Can you work these out from the drawing? Everything is in mm from the part's minimum corner. A direction names the side the tool comes from. Coordinates: 2 decimals unless noted, no trailing zeros. Loops run counter-clockwise (first coordinate to the right, second up) from the corner with the lowest first, then second, coordinate; pieces in that order, holes last.
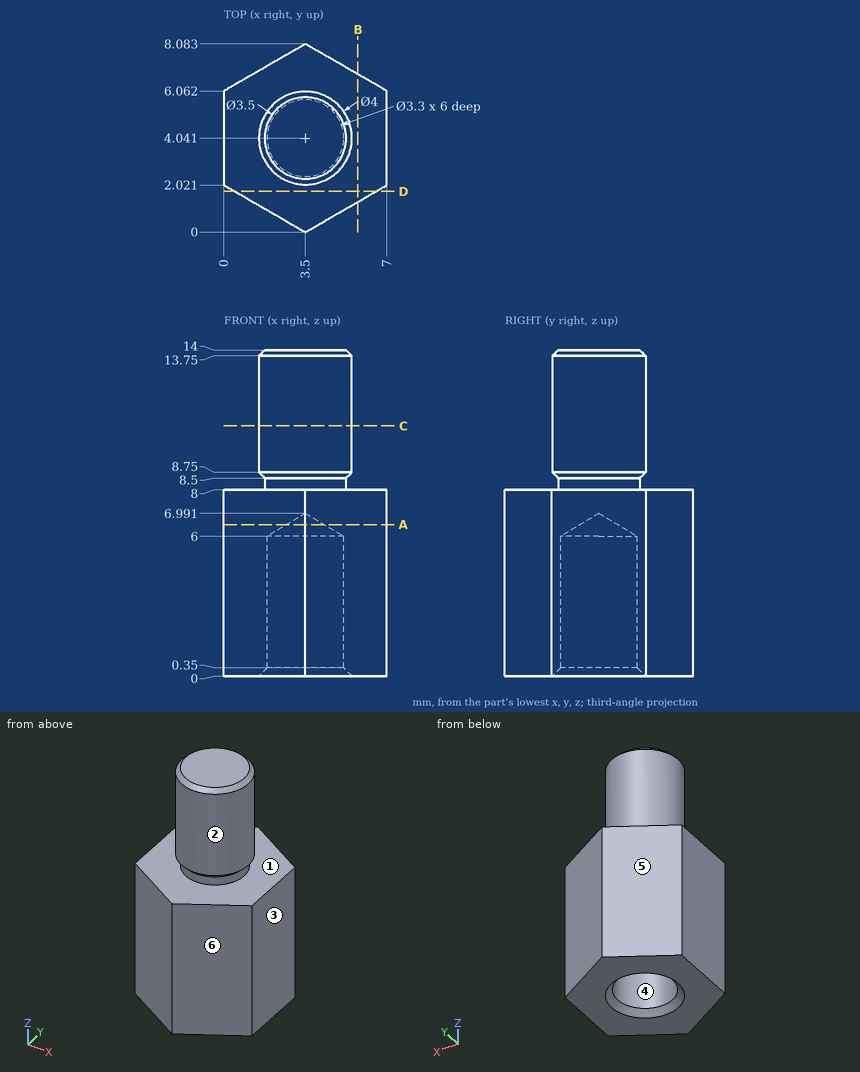
1) Imagine slicing it at C-C on z = 10.75. List the corners of the cut face in (x, y) for me, plus the area to 3 significant figures.
2) Imagine slicing it at A-A on z = 6.5. List the corners of the cut face in (x, y) for me (1 decimal).
3) Imagine slicing it at B-B on x = 5.75. List the corners of the cut face in (y, z) for me.
4) Imagine slicing it at D-D on y = 1.75. List the corners of the cut face in (x, z) for me.
5) For the marked faces 1, 2 and 3, which set-ups out of +Z, -Z, +X, -X, +Y, -Y let a thin tool reach every point of the face, with its end or its side?
6) If I drill on L1, parallel to Z at x = 6.5, y = 4.25; L2, parallel to Y at x = 3, z = 4.5 (1 decimal); L3, parallel to X at y = 4, z = 6.5 (1 decimal), over which ranges is the centre line in solid material (lowest first)?
7) We'd pull the mould along Y, two halves only. Please class the marked faces 4, 5 and 6: released by +Y, released by -Y, zero draft, split by the parting line, or undercut.
8) Will these pins go through, and if not, where does the flat tip stop? pin 1 (3 mm diameter, centred on y = 1, z = 12.5, fed in from +X) (1 decimal); pin 2 (1.1 mm diameter, centred on x = 3, y = 4.5, fed in from -Z); pin 3 (2 mm diameter, centred on y = 3, z = 10, fed in from +X).
Solved:
1. outline: circle Ø4 at (3.5, 4.04)
1. area: 12.6 mm2
2. outline: (0, 2) - (3.5, 0) - (7, 2) - (7, 6.1) - (3.5, 8.1) - (0, 6.1) - close; hole circle Ø1.6 at (3.5, 4)
3. outline: (1.3, 0) - (6.78, 0) - (6.78, 8) - (1.3, 8) - close
4. outline: (0.47, 0) - (6.53, 0) - (6.53, 8) - (0.47, 8) - close
5. face 1: none
5. face 2: +Z
5. face 3: +Z, -Z, +X, +Y, -Y
6. L1: z = 0 to 8
6. L2: y = 0.3 to 2.5, 5.6 to 7.8
6. L3: x = 0 to 2.7, 4.3 to 7
7. face 4: undercut
7. face 5: released by +Y
7. face 6: released by -Y
8. pin 1: stops at x = 4.8
8. pin 2: stops at z = 6.25
8. pin 3: stops at x = 5.5
